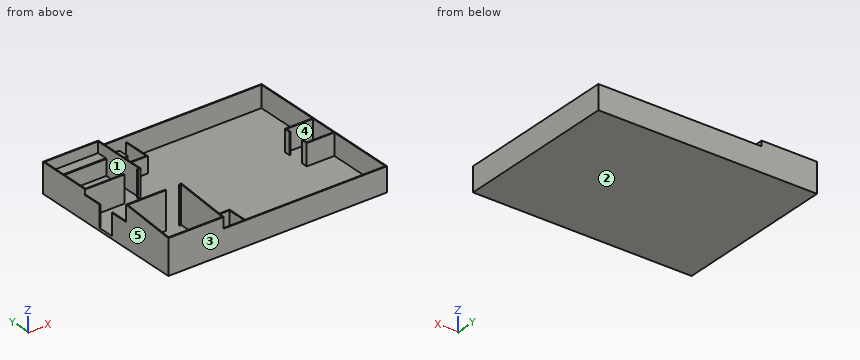
```python
from build123d import *

# Parameters (mm, degrees)
F0_W         = 103.7166666667
F0_H         = 77.8933333333
F1_DEPTH     = 1.27
F2_W         = 102.87
F2_H         = 0.4233333333
F2_W_2       = 0.4233333333
F3_DEPTH     = 10.16
F4_W         = 25.4
F4_H         = 25.4
F5_DEPTH     = 2.54
F6_W         = 25.4
F6_H         = 5.08
F7_DEPTH     = 7.62
F8_SIZE      = 0.254
F10_DEPTH    = 17.78
F12_DEPTH    = 7.62
F14_DEPTH    = 10.16
F15_T1_DEPTH = 162.7058608064
F16_W        = 11.0460426462
F16_H        = 7.62
F16_W_2      = 6.35
F16_H_2      = 7.8945169225
F16_H_3      = 7.643327117
F17_DEPTH    = 25.4
F19_DEPTH    = 7.62
F18_R        = 0.635
F20_ANGLE    = 90
F21_W        = 8.89
F21_H        = 5.08
F22_DEPTH    = 5.08
F23_DEPTH    = 2.54


# Not quite as in the source:
# - a fillet or chamfer that OpenCascade refuses, or shapes differently, is made with other operations: its cross-section is extruded or revolved along the edge and cut away or added


with BuildPart() as f1:
    # F0 (on Top) → F1 (new body)
    with BuildSketch(Plane.XY):
        Rectangle(F0_W, F0_H)
    extrude(amount=F1_DEPTH)

    # F2 (on face) → F3 (join)
    with BuildSketch(Plane.XY.offset(1.27)):
        Polygon((-25.6116666667, 38.5233333333), (-26.035, 38.5233333333), (-26.035, 13.1233333333), (-51.435, 13.1233333333), (-51.435, 12.7), (-25.6116666667, 12.7), align=None)
        Polygon((-51.435, 13.1233333333), (-51.435, 38.5233333333), (-26.035, 38.5233333333), (-25.6116666667, 38.5233333333), (38.6280342937, 38.5233333333), (51.435, 38.5233333333), (51.8583333333, 38.5233333333), (51.8583333333, 38.9466666667), (-51.8583333333, 38.9466666667), (-51.8583333333, -38.5233333333), (-51.435, -38.5233333333), (-51.435, -30.5099412799), (-51.435, 12.7), align=None)
        Polygon((51.8583333333, 38.5233333333), (51.435, 38.5233333333), (51.435, -38.5233333333), (51.435, -38.9466666667), (51.8583333333, -38.9466666667), align=None)
        with Locations((0, -38.735)):
            Rectangle(F2_W, F2_H)
        with Locations((-51.6466666667, -38.735)):
            Rectangle(F2_W_2, F2_H)
    extrude(amount=F3_DEPTH)

    # F4 (on face) → F5 (join)
    with BuildSketch(Plane.XY.offset(11.43)):
        Polygon((-25.6116666667, 12.7), (-25.6116666667, 38.5233333333), (-25.6116666667, 38.9466666667), (-51.8583333333, 38.9466666667), (-51.8583333333, 12.7), (-51.435, 12.7), align=None)
        with Locations((-38.735, 25.8233333333)):
            Rectangle(F4_W, F4_H, mode=Mode.SUBTRACT)
    extrude(amount=F5_DEPTH)

    # F6 (on face) → F7 (join)
    with BuildSketch(Plane.XY.offset(1.27)):
        with Locations((-38.735, 35.9833333333)):
            Rectangle(F6_W, F6_H)
    extrude(amount=F7_DEPTH)

    # F8
    f8_edges = [f1.edges().sort_by_distance(p)[0] for p in [
        (-38.735, 33.443333, 8.89),
    ]]
    chamfer(f8_edges, length=F8_SIZE)

    # F9 (on face) → F10 (join)
    with BuildSketch(Plane.XY.offset(1.27)):
        Polygon((-26.035, -13.1233333333), (-26.035, -38.5233333333), (-25.6116666667, -38.5233333333), (-25.6116666667, -12.7), (-51.435, -12.7), (-51.435, -13.1233333333), align=None)
    extrude(amount=F10_DEPTH)

    # F11 (on face) → F12 (join)
    with BuildSketch(Plane.XY.offset(11.43)):
        Polygon((-25.6116666667, -38.9466666667), (-25.6116666667, -38.5233333333), (-26.035, -38.5233333333), (-51.435, -38.5233333333), (-51.435, -13.1233333333), (-51.435, -12.7), (-51.8583333333, -12.7), (-51.8583333333, -38.9466666667), align=None)
    extrude(amount=F12_DEPTH)

    # F13 (on face) → F14 (join)
    with BuildSketch(Plane.XY.offset(1.27)):
        Polygon((51.435, -6.7733333333), (51.435, -6.35), (38.735, -6.35), (38.735, -3.81), (38.3116666667, -3.81), (38.3116666667, -6.7733333333), align=None)
        Polygon((38.735, 6.35), (51.435, 6.35), (51.435, 6.7733333333), (38.3116666667, 6.7733333333), (38.3116666667, 3.81), (38.735, 3.81), align=None)
    extrude(amount=F14_DEPTH)

    # F15: chamfer of 2.54 x 26.2466666667 on 1 edges, made by hand

    # F15_s2 → F15_t1 (cut)
    with BuildSketch(Plane.YZ.offset(-120.0879304032)):
        Polygon((-12.7, 19.05), (-38.9466666667, 16.51), (-38.9466666667, 19.05), align=None)
    extrude(amount=F15_T1_DEPTH, mode=Mode.SUBTRACT)

    # F16 (on face) → F17 (cut)
    with BuildSketch(Plane.XY.offset(1.27)):
        with Locations((-51.2559060007, 0)):
            Rectangle(F16_W, F16_H)
        with Locations((-30.0566666667, 11.1596328206)):
            Rectangle(F16_W_2, F16_H_2)
        with Locations((-30.0566666667, -12.5059764832)):
            Rectangle(F16_W_2, F16_H_3)
    extrude(amount=F17_DEPTH, mode=Mode.SUBTRACT)

    # F18 (on face) → F19 (join)
    with BuildSketch(Plane.XY.offset(1.27)):
        Polygon((-12.4883333333, 38.5233333333), (-12.9116666667, 38.5233333333), (-12.9116666667, 25.8233333333), (-25.6116666667, 25.8233333333), (-25.6116666667, 25.4), (-12.4883333333, 25.4), align=None)
        Polygon((-12.9116666667, -38.5233333333), (-12.4883333333, -38.5233333333), (-12.4883333333, -25.4), (-25.6116666667, -25.4), (-25.6116666667, -25.8233333333), (-12.9116666667, -25.8233333333), align=None)
    extrude(amount=F19_DEPTH)

    # F18 (on face) → F20 (revolve)
    with BuildSketch(Plane.XY.offset(1.27)):
        with Locations((-14.3933333333, 37.0416666667)):
            Circle(F18_R)
        with Locations((-14.3933333333, -37.0416666667)):
            Circle(F18_R)
    revolve(axis=Axis((-15.4516666667, 37.5929450293, 1.27), (0, -1, 0)), revolution_arc=F20_ANGLE)

    # F21 (on face) → F22 (join)
    with BuildSketch(Plane.XY.offset(1.27)):
        with Locations((-20.32, 35.9833333333)):
            Rectangle(F21_W, F21_H)
        with Locations((-20.32, -35.9833333333)):
            Rectangle(F21_W, F21_H)
    extrude(amount=F22_DEPTH)

    # F23 (add): faces of the model
    f23_faces = [f1.faces().sort_by_distance(p)[0] for p in [
        (-15.4516666667, 37.0416666667, 2.3283333333),
        (-15.4516666667, -37.0416666667, 2.3283333333),
    ]]
    extrude(f23_faces, amount=F23_DEPTH)


solid = f1.part
```
For this review, take the finished solid that the model builds, in its own axes (mm). Face numbers are marked on the shaded views. A direction names the side the tool comes from. Round coordinates to 2 decimals unless told otherwise and drop trailing zeros. Write each loop counter-clockwise with the first axis right and the second up, starting at its lowest first coordinate (ties: lowest second). Pieces come first, ordered by that corner, then holes. Notation, with made-up numbers: (61, 30.5) -> (115, 30.5) arc R5 cw to (115, 37.5) -> close; hole circle Ø10 at (1, 24). An arc over 180 degrees is marked (long way). Use one line per item in the form item = value.
Q1. The part is to be moulded in two halves that separate along X. For the marked faces 3, 4 and 5, say which applies: released by +X, released by -X, zero draft, split by the parting line, or undercut.
Resolved:
face_3 = zero draft
face_4 = undercut
face_5 = released by -X
Q2. Consider section B-B (y = 29). State the section outline as (x, z) points (3 decimals).
Resolved:
outline = (-51.858, 0) -> (51.858, 0) -> (51.858, 11.43) -> (51.435, 11.43) -> (51.435, 1.27) -> (-12.488, 1.27) -> (-12.488, 8.89) -> (-12.912, 8.89) -> (-12.912, 1.27) -> (-25.612, 1.27) -> (-25.612, 13.97) -> (-26.035, 13.97) -> (-26.035, 1.27) -> (-51.435, 1.27) -> (-51.435, 13.97) -> (-51.858, 13.97) -> close
Q3. Consider section C-C (x = 44.5). State the section outline as (y, z) points.
Resolved:
outline = (-38.95, 0) -> (38.95, 0) -> (38.95, 11.43) -> (38.52, 11.43) -> (38.52, 1.27) -> (6.77, 1.27) -> (6.77, 11.43) -> (6.35, 11.43) -> (6.35, 1.27) -> (-6.35, 1.27) -> (-6.35, 11.43) -> (-6.77, 11.43) -> (-6.77, 1.27) -> (-38.52, 1.27) -> (-38.52, 11.43) -> (-38.95, 11.43) -> close
Q4. To check wall thickness, follow probe 1 along X at (y, z) = (-18.5, 2.25) (3 decimals); probe 2 along X at (y, z) = (-35, 7.5) (3 decimals); probe 3 along X at (y, z) = (-25.5, 6.5) (3 decimals). State the ranges of each line that lie inside material, in increasing order. Write a range as from..to.
Resolved:
probe_1 = -51.858..-51.435, -26.035..-25.612, 51.435..51.858
probe_2 = -51.858..-51.435, -26.035..-25.612, -12.912..-12.488, 51.435..51.858
probe_3 = -51.858..-51.435, -26.035..-12.488, 51.435..51.858
Q5. Clearance check with a flat-ended pin moving along its axis: pin 1 Ø1.5 at (x, y) = (-18.5, -37) entering from +Z. State where the tip first meets the part, or that it passes through.
Resolved:
pin_1 = 6.35
Q6. Machinability: for the marked faces 1 and 2, which of the approach directions +Z, -Z, +X, -X, +Y, -Y give a long, thin tool a straight path to every point of the face, cutting with its end or side? Answer none if there is none.
Resolved:
face_1 = +Z
face_2 = -Z, +X, -X, +Y, -Y
Q7. Consider section D-D (z = 4.75). State how many separate pieces and enclosed holes the cut face has, then the cut area to 3 significant figures.
Resolved:
separate_pieces = 1
enclosed_holes = 2
area = 442 mm²
Q8. Consider section A-A (z = 15.25). State the section outline as (x, y) points (3 decimals).
Resolved:
outline = (-51.858, -38.947) -> (-25.612, -38.947) -> (-25.612, -12.7) -> (-26.882, -12.7) -> (-26.882, -13.123) -> (-26.035, -13.123) -> (-26.035, -38.523) -> (-51.435, -38.523) -> (-51.435, -13.123) -> (-33.232, -13.123) -> (-33.232, -12.7) -> (-51.858, -12.7) -> close
